Autodesk Inventor part; units mm, degrees
ref_plane "YZ Plane" through (0, 0, 0) normal (1, 0, 0) x (0, 1, 0)
ref_plane "XZ Plane" through (0, 0, 0) normal (0, 1, 0) x (-1, 0, 0)
ref_plane "XY Plane" through (0, 0, 0) normal (0, 0, 1) x (1, 0, 0)
sketch "Szkic1" plane through (0, 0, 0) normal (0, 1, 0) x (-1, 0, 0)
  line L0 (2.5, -45) -> (-2.5, -45)
  line L1 (-7.5, -40) -> (-7.5, 40)
  line L2 (-2.5, 45) -> (2.5, 45)
  line L3 (7.5, 40) -> (7.5, -40)
  line L4 (7.5, -45) -> (-7.5, 45) construction
  line L5 (-7.5, -45) -> (7.5, 45) construction
  arc A0 (7.5, 40) -> (2.5, 45) centre (2.5, 40) ccw
  arc A1 (-2.5, 45) -> (-7.5, 40) centre (-2.5, 40) ccw
  arc A2 (2.5, -45) -> (7.5, -40) centre (2.5, -40) ccw
  arc A3 (-7.5, -40) -> (-2.5, -45) centre (-2.5, -40) ccw
  circle A4 centre (0, 40) radius 2
  circle A5 centre (0, -10) radius 2
  circle A6 centre (0, -40) radius 2
  point P0 (0, 0)
  dimension "d0" = 15
  dimension "d1" = 90
  dimension "d2" = 5
  dimension "d3" = 4
  dimension "d4" = 4
  dimension "d5" = 4
extrude "Wyciągnięcie proste1" add sketch "Szkic1" along normal blind 6
properties part number "ArmLifter"
Verification items for the finished model (mm, model axes). Round coordinates to 2 decimals unless told otherwise and drop trailing zeros. Order: outer loops, then holes, each group sorted by start corner. A loop starts at its lowest first (then second) coordinate and runs counter-clockwise, first axis right, second up.
1) Cross-section at B-B, the plane y = 0.75. Record the cut outline in (x, z), plus the area to 3 significant figures.
Geometry says:
outline: (-7.5, -40) arc R5 ccw to (-2.5, -45) - (2.5, -45) arc R5 ccw to (7.5, -40) - (7.5, 40) arc R5 ccw to (2.5, 45) - (-2.5, 45) arc R5 ccw to (-7.5, 40) - close; hole circle Ø4 at (0, -40); hole circle Ø4 at (0, -10); hole circle Ø4 at (0, 40)
area: 1,290 mm2
2) Cross-section at A-A, the plane z = -10. Record the cut outline in (x, y).
Geometry says:
outline: (-7.5, 0) - (-2, 0) - (-2, 6) - (-7.5, 6) - close; (2, 0) - (7.5, 0) - (7.5, 6) - (2, 6) - close
3) Cross-section at C-C, the plane x = 0. Record the cut outline in (y, z).
Geometry says:
outline: (0, -45) - (6, -45) - (6, -42) - (0, -42) - close; (0, -38) - (6, -38) - (6, -12) - (0, -12) - close; (0, -8) - (6, -8) - (6, 38) - (0, 38) - close; (0, 42) - (6, 42) - (6, 45) - (0, 45) - close
4) Draft check along X on faces 1 (the flat face through (0, 0, 1)), 2 (the cylindrical face through (0, 3, 42)), 3 (the cylindrical face through (-6.07, 2.96, -43.5)). Enter one of: +X half, -X half, draft (parallel to the pull), parting line (faces both ways), or undercut.
Geometry says:
face 1: draft
face 2: undercut
face 3: -X half
5) Material ranges on line 1 (Z direction, x = 0, y = 4.5); line 2 (Z direction, x = 6, y = 5.6); line 3 (Z direction, x = 4.25, y = 1.45), recorded low to high.
Geometry says:
line 1: z = -45 to -42, -38 to -12, -8 to 38, 42 to 45
line 2: z = -43.57 to 43.57
line 3: z = -44.68 to 44.68
6) Cross-section at D-D, the plane x = -5.5. Record the cut outline in (y, z), plus the area to 3 significant figures.
Geometry says:
outline: (0, -44) - (6, -44) - (6, 44) - (0, 44) - close
area: 528 mm2
